Could you check a few things on this model? Use its own coordinates, in mm. Round coordinates to 2 decimals unless told otherwise and drop trailing zeros. Write each loop counter-clockwise with the first axis right and the second up, starting at its lowest first coordinate (ties: lowest second). Pieces come first, ordered by that corner, then holes. Notation, with made-up numbers: M -31.75,-35.5 L 12.25,-35.5 A15 cw 12.25,-22.5 Z; hole C 10,83 d2. An arc over 180 degrees is marked long. One line per item, written item: value. Start each with the question number.
(1) I want a section at C-C on x = 0. Please give me the cut outline in (y, z), and give its area (3 significant figures).
(2) Thinking about a two-plate mould opening in X: for faces 1 (the face through (-4.88, 2.96, -1.08)), 2 (the face through (0, 0, 0)), which applies, released by +X, released by -X, zero draft, split by the parting line, or undercut?
(3) I want a section at D-D on z = 3. Please give me the cut outline in (x, y).
(4) I'm going to push flat-ended pins straight in: pin 1 Ø5 at (y, z) = (9, 0.5) entering from -X; pin 2 Ø6 at (y, z) = (6.5, -3.5) entering from -X; pin 3 Ø5 at (x, z) = (1, -2.5) entering from +Y. Where does each tip first touch, or does it pass through?
(5) If I drill on L1, parallel to Y at x = 2.75, z = 1; L2, parallel to X at y = 7.25, z = 0; L3, parallel to X at y = 4, z = -1.75, over which ranges is the centre line in solid material (lowest first)?
(6) I want a section at B-B on z = 0. Please give me the cut outline in (x, y).
(7) I want a section at A-A on y = 8.75. Please give me the cut outline in (x, z).
```python
from build123d import *

# Parameters (mm, degrees)
SKETCH_1_R      = 5
EXTRUDE_1_DEPTH = 6
SKETCH_2_R      = 0.25
EXTRUDE_2_DEPTH = 6


with BuildPart() as part:
    # Эскиз1 → Бобышка-Вытянуть1 (new body)
    with BuildSketch(Plane(origin=(0, 0, 0), x_dir=(1, 0, 0), z_dir=(0, 1, 0))):
        with Locations(Location((0, 0, 0), (0, 0, 270))):
            Circle(SKETCH_1_R)
    extrude(amount=EXTRUDE_1_DEPTH)

    # Эскиз2 → Бобышка-Вытянуть2 (add)
    with BuildSketch(Plane(origin=(0, 6, 0), x_dir=(1, 0, 0), z_dir=(0, 1, 0))):
        with Locations(Location((-2.5, 0, 0), (0, 0, 270))):
            Circle(SKETCH_2_R)
        with Locations(Location((2.5, 0, 0), (0, 0, 90))):
            Circle(SKETCH_2_R)
    extrude(amount=EXTRUDE_2_DEPTH)


solid = part.part
```
Found:
1. outline: M 0,-5 L 6,-5 L 6,5 L 0,5 Z
1. area: 60.0 mm²
2. face 1: split by the parting line
2. face 2: zero draft
3. outline: M -4,0 L 4,0 L 4,6 L -4,6 Z
4. pin 1: stops at x = -2.75
4. pin 2: stops at x = -4.97
4. pin 3: stops at y = 6
5. L1: y = 0 to 6
5. L2: x = -2.75 to -2.25, 2.25 to 2.75
5. L3: x = -4.68 to 4.68
6. outline: M -5,0 L 5,0 L 5,6 L 2.75,6 L 2.75,12 L 2.25,12 L 2.25,6 L -2.25,6 L -2.25,12 L -2.75,12 L -2.75,6 L -5,6 Z
7. outline: C -2.5,0 d0.5; C 2.5,0 d0.5
